Source: three-view drawing plus pictorial views. Frame: mm from the lowest corner of the part. Give positions to 0.01 mm unless a question says otherwise; leave off trailing zeros. Loops run counter-clockwise (first coordinate to the right, second up) from the corner with the lowest first, then second, coordinate; pieces in that order, holes last. Notation, with made-up numbers: (9.25, 23) - (58.25, 23) arc R28 cw to (58.25, 49) - close; hole circle Ø8 at (85.5, 37.5). An arc over 180 degrees is marked (long way). Answer as a JSON object with one key per item and string values.
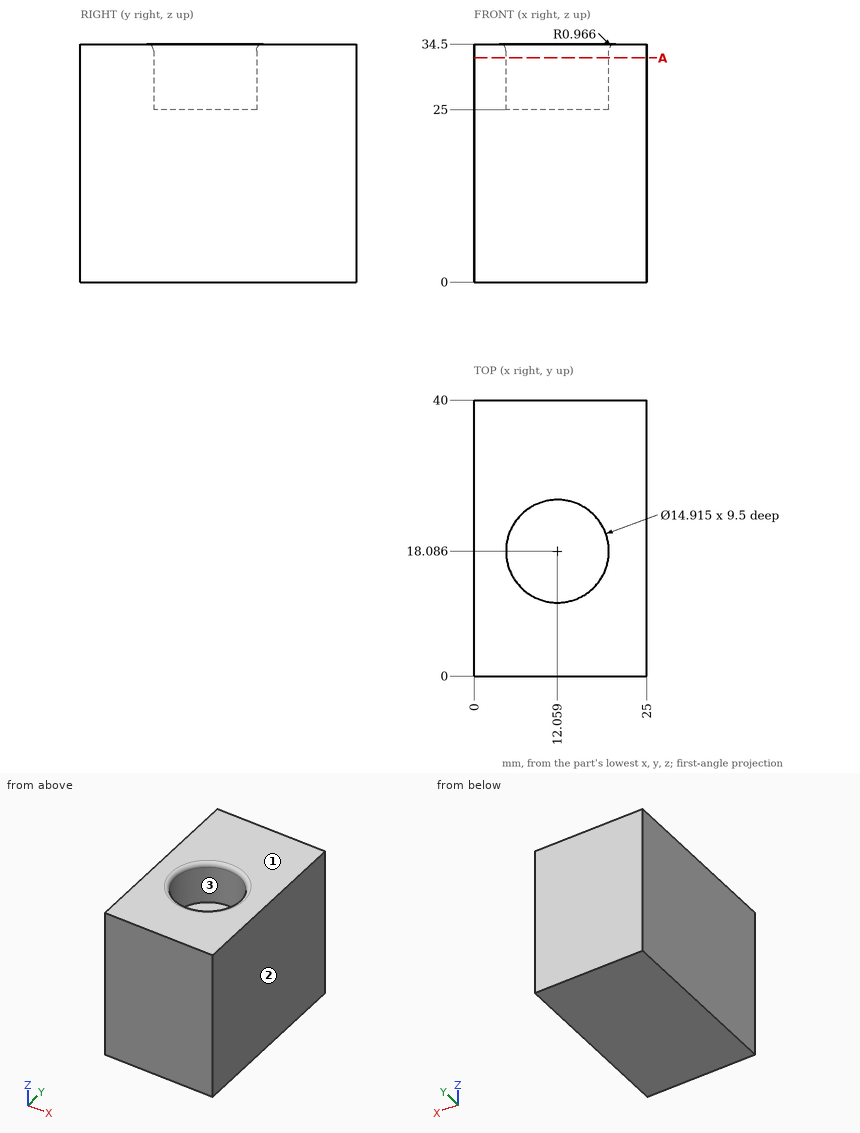
Item 1: Cut plane A-A (z = 32.5). Return loops of the section in (x, y) (1 decimal).
Geometry check:
{"outline": "(0, 0) - (25, 0) - (25, 40) - (0, 40) - close; hole circle Ø14.9 at (12.1, 18.1)"}
Item 2: Material intervals for line 1 (Z direction, x = 13.25, y = 25); line 2 (X direction, y = 15, z = 32); line 3 (X direction, y = 25, z = 27) (1 decimal), sorted ascending. Write a range as [from, to].
Geometry check:
{"line 1": "z = [0, 25]", "line 2": "x = [0, 5.27], [18.85, 25]", "line 3": "x = [0, 9.3], [14.9, 25]"}
Item 3: Mould query, pull axis X, two halves, no side actions, for the marked faces 1, 2 and 3. Classes: released by +X, released by -X, zero draft, split by the parting line, or undercut.
Geometry check:
{"face 1": "zero draft", "face 2": "released by +X", "face 3": "undercut"}
Item 4: Contact query for a flat-ended pin moving along its axis: P1, Ø4.5, axis at x = 14.5, y = 20, coming from the +Z side. Output: stop coordinate, or through.
Geometry check:
{"P1": "stops at z = 25"}
